CAD build for the part. Positions are in the model's coordinates, mm. A direction names the side the tool comes from. Coordinates: 2 decimals unless noted, no trailing zeros. Order: outer loops, then holes, each group sorted by start corner. A loop starts at its lowest first (then second) coordinate and runs counter-clockwise, first axis right, second up. Notation, with made-up numbers: (-14, 75) - (40, 75) arc R4 ccw to (40, 80) - close; hole circle Ø2 at (73.5, 47.25). An arc over 180 degrees is marked (long way). Return JSON: item names as keys, results as strings.
from build123d import *

# Parameters (mm, degrees)
SALIENTE_EXTRUIR1_DEPTH = 18
SALIENTE_EXTRUIR2_DEPTH = 7
CROQUIS4_W              = 22
CROQUIS4_H              = 4.8
SALIENTE_EXTRUIR3_DEPTH = 10
REDONDEO1_R             = 10
REDONDEO2_R             = 3
CROQUIS5_R              = 1.5
CORTAR_EXTRUIR1_DEPTH   = 104.776547512
CROQUIS6_W              = 40
CROQUIS6_H              = 15
SALIENTE_EXTRUIR4_DEPTH = 5
REDONDEO3_R             = 10
REDONDEO4_R             = 15
REDONDEO5_R             = 2


with BuildPart() as part:
    # Croquis1 → Saliente-Extruir1 (new body)
    with BuildSketch(Plane(origin=(0, 0, 0), x_dir=(1, 0, 0), z_dir=(0, 1, 0))):
        with BuildLine():
            Line((-20.173769885, -4.363411025), (-17.4, -9.8))
            Line((-17.4, -9.8), (-17.4, -10.3))
            Line((-17.4, -10.3), (17.4, -10.3))
            Line((17.4, -10.3), (17.4, -9.8))
            Line((17.4, -9.8), (20.173769885, -4.363411025))
            ThreePointArc((20.173769885, -4.363411025), (20.059826813, -1.433193227), (17.501484276, 0))
            Line((17.501484276, 0), (-17.501484276, 0))
            ThreePointArc((-17.501484276, 0), (-20.059826813, -1.433193227), (-20.173769885, -4.363411025))
        make_face()
    extrude(amount=SALIENTE_EXTRUIR1_DEPTH)

    # Croquis2 → Saliente-Extruir2 (add)
    with BuildSketch(Plane.XY.offset(10.3)):
        with BuildLine():
            Line((-17.4, 18), (-23.118519933, 18))
            ThreePointArc((-23.118519933, 18), (-31.310040375, 13.735764364), (-32.51544614, 4.579798567))
            Line((-32.51544614, 4.579798567), (-6.462530087, -67))
            Line((-6.462530087, -67), (67.195200278, -40.190778624))
            ThreePointArc((67.195200278, -40.190778624), (86.478828568, -6.79055467), (56.934595978, 18))
            Line((56.934595978, 18), (-17.4, 18))
        make_face()
    extrude(amount=SALIENTE_EXTRUIR2_DEPTH)

    # Croquis4 → Saliente-Extruir3 (add)
    with BuildSketch(Plane(origin=(-27.239942599, -9.914528289, 0), x_dir=(0, 0, 1), z_dir=(-0.939692620785908, -0.3420201433256697, 0))):
        with Locations((28.3, -49.249090126)):
            Rectangle(CROQUIS4_W, CROQUIS4_H)
    extrude(amount=-SALIENTE_EXTRUIR3_DEPTH)

    # Redondeo1
    # the kernel refuses this fillet: 10 mm, written as the material it adds along each edge
    with BuildSketch(Plane(origin=(-9.574913392, -58.448797151, 17.3), x_dir=(0.3420201433256697, -0.939692620785908, -1.1712242897144546e-15), z_dir=(0.9396926207859081, 0.34202014332566977, 0))) as redondeo1_piece_1:
        with BuildLine():
            CenterArc((10, -9.959417654), REDONDEO1_R, 95.163607091, 84.836392909)
            Line((0, -9.959417654), (-0.2, -9.959417654))
            Line((-0.2, -9.959417654), (-0.2, 0))
            Line((-0.2, 0), (0, 0.2))
            ThreePointArc((0, 0.2), (4.55, 0.2), (9.082, 0.199188353))
            Line((9.082, 0.199188353), (9.1, 0))
        make_face()
    extrude(amount=10)
    with BuildSketch(Plane(origin=(-11.21661008, -53.938272571, 17.3), x_dir=(-0.3420201433256697, 0.939692620785908, 0), z_dir=(0.9396926207859081, 0.34202014332566977, 0))) as redondeo1_piece_2:
        with BuildLine():
            CenterArc((REDONDEO1_R, REDONDEO1_R), REDONDEO1_R, 180, 90)
            Line((0, REDONDEO1_R), (-REDONDEO1_R * 0.02, REDONDEO1_R))
            Line((-REDONDEO1_R * 0.02, REDONDEO1_R), (-REDONDEO1_R * 0.02, -REDONDEO1_R * 0.02))
            Line((-REDONDEO1_R * 0.02, -REDONDEO1_R * 0.02), (REDONDEO1_R, -REDONDEO1_R * 0.02))
            Line((REDONDEO1_R, -REDONDEO1_R * 0.02), (REDONDEO1_R, 0))
        make_face()
    extrude(amount=10)

    # Redondeo2
    redondeo2_edges = [part.edges().sort_by_distance(p)[0] for p in [
        (-0.998835528, -52.773333428, 39.3),
        (-10.395761736, -56.193534861, 39.3),
    ]]
    fillet(redondeo2_edges, radius=REDONDEO2_R)

    # Croquis5 → Cortar-Extruir1 (cut, through all)
    with BuildSketch(Plane(origin=(17.665029208, -48.534268862, 0), x_dir=(0.9396926207859081, 0.34202014332566977, 0), z_dir=(0.3420201433256697, -0.939692620785908, 0))):
        with Locations((-23.988141438, 35.3)):
            Circle(CROQUIS5_R)
    extrude(amount=-CORTAR_EXTRUIR1_DEPTH, mode=Mode.SUBTRACT)

    # Croquis6 → Saliente-Extruir4 (add)
    with BuildSketch(Plane(origin=(20.777412512, -57.085471711, 0), x_dir=(0.9396926207859081, 0.3420201433256697, 0), z_dir=(0.34202014332566966, -0.939692620785908, 0))):
        with Locations((1.011858562, 24.8)):
            Rectangle(CROQUIS6_W, CROQUIS6_H)
    extrude(amount=-SALIENTE_EXTRUIR4_DEPTH)

    # Redondeo3
    redondeo3_edges = [part.edges().sort_by_distance(p)[0] for p in [
        (2.079345762, -61.230567015, 32.3),
        (39.667050594, -47.549761282, 32.3),
    ]]
    fillet(redondeo3_edges, radius=REDONDEO3_R)

    # Redondeo4
    # the kernel refuses this fillet: 15 mm, written as the material it adds along each edge
    with BuildSketch(Plane(origin=(40.522100952, -49.898992834, 17.3), x_dir=(-0.08679417196563514, -0.03159049510327337, 0.9957252695055648), z_dir=(-0.3420201433256697, 0.9396926207859082, 0))) as redondeo4_piece_1:
        with BuildLine():
            CenterArc((13.743188401, 14.243145828), REDONDEO4_R, 185.299645608, 66.421821522)
            Line((-1.192690642, 12.857679399), (-2.686278546, 12.719132757))
            Line((-2.686278546, 12.719132757), (-1.493587904, -0.138546643))
            Line((-1.493587904, -0.138546643), (0.138546643, -1.493587904))
            ThreePointArc((0.138546643, -1.493587904), (5.11717299, -1.031765761), (8.568182674, -1.424314583))
            Line((8.568182674, -1.424314583), (9.03863774, 0))
        make_face()
    extrude(amount=5)

    # Redondeo5
    redondeo5_edges = [part.edges().sort_by_distance(p)[0] for p in [
        (37.167297989, 18, 10.3),
        (-20.259259966, 18, 10.3),
        (-31.310040375, 13.735764364, 10.3),
        (-19.488988114, -31.210100717, 10.3),
        (30.366335095, -53.595389312, 10.3),
        (86.478828568, -6.79055467, 10.3),
    ]]
    fillet(redondeo5_edges, radius=REDONDEO5_R)


solid = part.part
Item 1: Band-saw the part on A-A, the plane z = 30. List the corners of the cut face in (x, y).
Findings below:
{"outline": "(-11.22, -53.94) - (-9.57, -58.45) - (-0.18, -55.03) - (-1.82, -50.52) - close; (4.63, -57.64) - (6.34, -62.34) - (37.12, -51.14) - (35.41, -46.44) - close"}
Item 2: Wall check: L1, parallel to Z at x = 23, y = -31; L2, parallel to Z at x = -16.5, y = 4; L3, parallel to Y at x = 25, z = 30. Give the ranges that are in metal, low to high. Write a range as [from, to].
Findings below:
{"L1": "z = [10.3, 17.3]", "L2": "z = [0, 17.3]", "L3": "y = [-55.55, -50.23]"}
Item 3: Band-saw the part on B-B, the plane z = 7. List the corners of the cut face in (x, y).
Findings below:
{"outline": "(-18.83, 0) - (18.83, 0) - (18.83, 18) - (-18.83, 18) - close"}
Item 4: Drop flat-ended pins along their axis: P1, Ø0.8, axis at y = 9, z = 10.5, coming from the +X side; P2, Ø1.5, axis at x = 5.5, y = -29, coming from the +Z side; P3, Ø5, axis at y = -23, z = 8.5, coming from the +X side. Give the stop position or say it passes through.
Findings below:
{"P1": "stops at x = 77.68", "P2": "stops at z = 17.3", "P3": "stops at x = 84.51"}
Item 5: Which spindle directions (+Z, -Z, +X, -X, +Y, -Y) get a long thin tool onto all of the face, cutting with end or side? Do faces 4 (the flat face through (0, 0, 5)), 5 (the flat face through (-6.58, -52.25, 33.22)), 6 (the flat face through (20.331, -51.927, 23.923)), 7 (the flat face through (2.09, -61.26, 19.76)), 8 (the flat face through (18.767, 8.874, 7.12)). Say none if no direction does.
Findings below:
{"face 4": "-Z, +X, -X, -Y", "face 5": "+Z, -X, +Y", "face 6": "+Z, +Y", "face 7": "+Z, -Y", "face 8": "+X, +Y, -Y"}
Item 6: Mould opens along X. For faces 1 (the cylindrical face through (4.747, -60.222, 29.293)), 2 (the cylindrical face through (-18.77, -31.52, 10.9)), 3 (the cylindrical face through (20.1, 8.9, 1.5)) say: released by +X, released by -X, zero draft, split by the parting line, or undercut.
Findings below:
{"face 1": "undercut", "face 2": "released by -X", "face 3": "released by +X"}
